Design review of the part built by this model. Coordinates are the model's own, in mm. A direction names the side the tool comes from. Round coordinates to 2 decimals unless told otherwise and drop trailing zeros. Order: outer loops, then holes, each group sorted by start corner. A loop starts at its lowest first (then second) coordinate and runs counter-clockwise, first axis right, second up. Notation, with made-up numbers: M -14,5.25 L 41,5.25 A27 ccw 41,33.25 Z; hole C -37.75,8.25 d2. An arc over 180 degrees is marked long. Write each question's results on one line, items separated by ' | '. Start each with the question number.
Item 1: Take a section at A-A, the plane y = 25.4. Write out the cut boundary in (x, z) (3 decimals), plus the area to 3 significant figures.
Item 2: Take a section at C-C, the plane z = 17. Write out the cut boundary in (x, y) (3 decimals), plus the area to 3 significant figures.
Item 3: Machinability: for faces 1 (the cylindrical face through (-15.12, -11.59, -12.61)), 2 (the cylindrical face through (-27.78, -0.1, -22.27)), 3 (the flat face through (14, 0, -25.4)), which of the approach directions +Z, -Z, +X, -X, +Y, -Y give a long, thin tool a straight path to every point of the face, cutting with its end or side? Answer none if there is none.
Item 4: The part is to be moulded in two halves that separate along Y. For faces 4 (the cylindrical face through (-2.75, 12.4, -5.05)), 5 (the cylindrical face through (-6.883, 30.995, 4.785)), 6 (the flat face through (14, 14, -3.175)), 7 (the cylindrical face through (-0.69, -3.1, 20.7)), say which applies: +Y half, -Y half, draft (parallel to the pull), parting line (faces both ways), or undercut.
Item 5: Clearance check with flat-ended pins moving along their axes: pin 1 (23 mm diameter, centred on x = 0, y = 0, fed in from -Z) (3 decimals); pin 2 (2 mm diameter, centred on y = 10.5, z = 2, fed in from +X); pin 3 (1 mm diameter, centred on y = 5, z = -15, fed in from -X). State where each tip first meets the part, or that it passes through.
Item 6: Take a section at D-D, the plane y = 0. Count the separate pieces of the cut face and the enclosed holes in it, plus the area to 3 significant figures.
Item 7: Wall thickness on line 1 (Y direction, x = 0, z = -23); line 2 (Z direction, x = -23, y = -4.5) (3 decimals): over which ranges is each line inside the solid? List them lowest first. Write a range as [from, to].
```python
from build123d import *

# Parameters (mm, degrees)
F0_R          = 19.05
F1_DEPTH      = 25.4
F1_DEPTH_BACK = 25.4
F2_R          = 31.75
F2_R_2        = 2.38125
F2_R_3        = 19.05
F3_DEPTH      = 6.35
F4_R          = 12.7
F5_DEPTH      = 41.275
F6_R          = 3.175
F7_DEPTH      = 9.525
F8_R          = 31.75
F8_R_2        = 19.05
F9_DEPTH      = 3.175
F13_R         = 31.75
F13_R_2       = 12.7
F14_DEPTH     = 3.175
F15_R         = 31.75
F15_R_2       = 12.7
F16_DEPTH     = 3.175
F17_R         = 31.75
F17_R_2       = 12.7
F18_DEPTH     = 3.175


with BuildPart() as f1:
    # F0 (on Top) → F1 (new body, two sides)
    with BuildSketch(Plane.XY) as f1_sk:
        Circle(F0_R)
    extrude(amount=F1_DEPTH)
    extrude(f1_sk.sketch, amount=-F1_DEPTH_BACK)

    # F2 (on face) → F3 (join)
    with BuildSketch(Plane(origin=(0, 0, -25.4), x_dir=(1, 0, 0), z_dir=(0, 0, -1))):
        Circle(F2_R)
        with Locations((0, -25.4)):
            Circle(F2_R_2, mode=Mode.SUBTRACT)
        with Locations((-25.4, 0)):
            Circle(F2_R_2, mode=Mode.SUBTRACT)
        Circle(F2_R_3, mode=Mode.SUBTRACT)
        with Locations((25.4, 0)):
            Circle(F2_R_2, mode=Mode.SUBTRACT)
        with Locations((0, 25.4)):
            Circle(F2_R_2, mode=Mode.SUBTRACT)
    extrude(amount=-F3_DEPTH)

    # F4 (on face) → F5 (cut)
    with BuildSketch(Plane(origin=(0, 0, -25.4), x_dir=(1, 0, 0), z_dir=(0, 0, -1))):
        Circle(F4_R)
    extrude(amount=-F5_DEPTH, mode=Mode.SUBTRACT)

    # F6 (on face) → F7 (cut)
    with BuildSketch(Plane.XY.offset(25.4)):
        Circle(F6_R)
    extrude(amount=-F7_DEPTH, mode=Mode.SUBTRACT)

    # F8 (on face) → F9 (join)
    with BuildSketch(Plane.XY.offset(25.4)):
        Circle(F8_R)
        Circle(F8_R_2, mode=Mode.SUBTRACT)
    extrude(amount=-F9_DEPTH)

    # F13 (on offset) → F14 (join)
    with BuildSketch(Plane(origin=(0, 0, 15.875), x_dir=(1, 0, 0), z_dir=(0, 0, -1))):
        Circle(F13_R)
        Circle(F13_R_2, mode=Mode.SUBTRACT)
    extrude(amount=F14_DEPTH)

    # F15 (on offset) → F16 (join)
    with BuildSketch(Plane(origin=(0, 0, 6.35), x_dir=(1, 0, 0), z_dir=(0, 0, -1))):
        Circle(F15_R)
        Circle(F15_R_2, mode=Mode.SUBTRACT)
    extrude(amount=F16_DEPTH)

    # F17 (on offset) → F18 (join)
    with BuildSketch(Plane(origin=(0, 0, -3.175), x_dir=(1, 0, 0), z_dir=(0, 0, -1))):
        Circle(F17_R)
        Circle(F17_R_2, mode=Mode.SUBTRACT)
    extrude(amount=F18_DEPTH)


solid = f1.part
```
Results list:
1) outline: M -19.05,-25.4 L -2.381,-25.4 L -2.381,-19.05 L -19.05,-19.05 Z; M -19.05,-6.35 L 19.05,-6.35 L 19.05,-3.175 L -19.05,-3.175 Z; M -19.05,3.175 L 19.05,3.175 L 19.05,6.35 L -19.05,6.35 Z; M -19.05,12.7 L 19.05,12.7 L 19.05,15.875 L -19.05,15.875 Z; M -19.05,22.225 L 19.05,22.225 L 19.05,25.4 L -19.05,25.4 Z; M 2.381,-25.4 L 19.05,-25.4 L 19.05,-19.05 L 2.381,-19.05 Z | area: 696 mm²
2) outline: C 0,0 d38.1; hole C 0,0 d6.35 | area: 1,110 mm²
3) face 1: none | face 2: -Z | face 3: -Z, +X, -X, +Y, -Y
4) face 4: undercut | face 5: parting line | face 6: draft | face 7: undercut
5) pin 1: z = 15.875 | pin 2: x = 16.51 | pin 3: x = -18.51
6) separate pieces: 4 | enclosed holes: 0 | area: 1,250 mm²
7) line 1: [-31.75, -27.78], [-23.02, -12.7], [12.7, 23.02], [27.78, 31.75] | line 2: [-25.4, -19.05], [-6.35, -3.175], [3.175, 6.35], [12.7, 15.875], [22.225, 25.4]
